Geometry: final body of the model. Coordinates: model frame, mm. Face numbers are marked on the shaded views. A direction names the side the tool comes from. Give positions to 0.01 mm unless a question says otherwise; leave off trailing zeros. Loops run counter-clockwise (first coordinate to the right, second up) from the corner with the lowest first, then second, coordinate; pieces in that order, holes last. Notation, with made-up numbers: M 12,15.5 L 33,15.5 A27 cw 33,54.5 Z; hole C 68.5,7.5 d3. An arc over 180 degrees is marked long. Put each result on its own line as item: value.
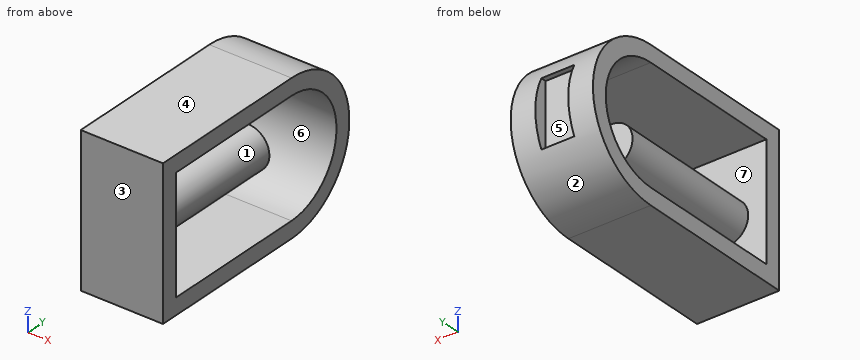
```python
from build123d import *

# Parameters (mm, degrees)
BOSS_EXTRUDE1_DEPTH = 127
SKETCH2_W           = 50.8
SKETCH2_H           = 101.6
CUT_EXTRUDE1_DEPTH  = 20.32
BOSS_EXTRUDE2_REACH = 351.192
SKETCH3_R           = 32.362244647


with BuildPart() as part:
    # Sketch1 → Boss-Extrude1 (new body)
    with BuildSketch(Plane(origin=(0, 0, 0), x_dir=(0, 0, -1), z_dir=(1, 0, 0))):
        with BuildLine():
            Line((-25.4, -25.4), (-25.4, 228.6))
            ThreePointArc((-25.4, 228.6), (88.9, 342.9), (203.2, 228.6))
            Line((203.2, 228.6), (203.2, -25.4))
            Line((203.2, -25.4), (-25.4, -25.4))
        make_face()
        with BuildLine():
            Line((0, 0), (177.8, 0))
            Line((177.8, 0), (177.8, 228.6))
            ThreePointArc((177.8, 228.6), (88.9, 317.5), (0, 228.6))
            Line((0, 228.6), (0, 0))
        make_face(mode=Mode.SUBTRACT)
    extrude(amount=BOSS_EXTRUDE1_DEPTH)

    # Sketch2 → Cut-Extrude1 (cut)
    with BuildSketch(Plane(origin=(0, 342.9, 0), x_dir=(1, 0, 0), z_dir=(0, 1, 0))):
        with Locations((63.5, 88.9)):
            Rectangle(SKETCH2_W, SKETCH2_H)
    extrude(amount=-CUT_EXTRUDE1_DEPTH, mode=Mode.SUBTRACT)

    # Sketch3 → Boss-Extrude2 (add, up to next)
    with BuildSketch(Plane(origin=(0, 228.6, 0), x_dir=(1, 0, 0), z_dir=(0, 1, 0)), mode=Mode.PRIVATE) as boss_extrude2_sk1:
        with Locations(Location((60.471295446, 97.62979548, 0), (0, 0, 270))):
            Circle(SKETCH3_R)
    boss_extrude2_tool1 = extrude(boss_extrude2_sk1.sketch, amount=-BOSS_EXTRUDE2_REACH, mode=Mode.PRIVATE) - part.part
    add(boss_extrude2_tool1.solids().sort_by_distance((60.471295, 228.6, -97.629795))[0])


solid = part.part
```
Item 1: Section A-A on y = 159. Output: boundary loops of the cut face in (x, z).
Output values:
outline: M 0,-203.2 L 127,-203.2 L 127,-177.8 L 0,-177.8 Z; M 0,0 L 127,0 L 127,25.4 L 0,25.4 Z; C 60.47,-97.63 d64.72
Item 2: Mould query, pull axis Z, two halves, no side actions, for the marked faces 1, 2 and 3. Classes: pulls with the +Z half, pulls with the -Z half, needs draft (parallel to the pull), parting line crosses it, or undercut.
Output values:
face 1: undercut
face 2: parting line crosses it
face 3: needs draft
Item 3: Section C-C on z = -86.5. Output: boundary loops of the cut face in (x, y), then the cut area to 3 significant figures.
Output values:
outline: M 0,-25.4 L 127,-25.4 L 127,0 L 90.86,0 L 90.86,228.6 L 30.08,228.6 L 30.08,0 L 0,0 Z; M 0,317.47 L 127,317.47 L 127,342.87 L 88.9,342.87 L 88.9,322.58 L 38.1,322.58 L 38.1,342.87 L 0,342.87 Z
area: 19,300 mm²
Item 4: Section B-B on x = 115.5. Output: boundary loops of the cut face in (y, z), then the cut area to 3 significant figures.
Output values:
outline: M -25.4,-203.2 L 228.6,-203.2 A114.3 ccw 228.6,25.4 L -25.4,25.4 Z; hole M 0,-177.8 L 228.6,-177.8 A88.9 ccw 228.6,0 L 0,0 Z
area: 25,500 mm²
Item 5: Pin query (flat end, axial travel): pin 1 Ø8 at (y, z) = (74, -0.5) entering from +X; pin 2 Ø1 at (y, z) = (227.5, -71.5) entering from +X; pin 3 Ø2.5 at (x, y) = (73.5, 325.5) entering from +Z; pin 4 Ø2 at (x, z) = (39, -106) entering from +Y. Return the tip coordinate at first contact, or that it passes through.
Output values:
pin 1: x = 127
pin 2: x = 80.23
pin 3: z = -26.33
pin 4: y = 341.68
Item 6: Line query: probe 1 along Y at (x, z) = (60, -91.5); probe 2 along Z at (x, y) = (115.5, 186.5); probe 3 along Z at (x, y) = (33, 165). Output: solid intervals per line, ascending. Write a range as [from, to].
Output values:
probe 1: [-25.4, 228.6], [317.46, 322.58]
probe 2: [-203.2, -177.8], [0, 25.4]
probe 3: [-203.2, -177.8], [-114.74, -80.52], [0, 25.4]
Item 7: Set-up query: the marked faces 4, 5, 6 and 7. Return all of +Z, -Z, +X, -X, +Y, -Y with unobstructed straight access to the full face (end or side cutting, diameter ignored); none if empty.
Output values:
face 4: +Z, +X, -X, +Y, -Y
face 5: +Y
face 6: +X, -X
face 7: none
Item 8: Section D-D on y = 268. Output: boundary loops of the cut face in (x, z), then the cut area to 3 significant figures.
Output values:
outline: M 0,-196.19 L 127,-196.19 L 127,-168.59 L 0,-168.59 Z; M 0,-9.21 L 127,-9.21 L 127,18.39 L 0,18.39 Z
area: 7,010 mm²
